The model under review builds one solid part; all positions refer to its coordinate system, in mm. Give positions to 0.01 mm unless a question says otherwise; leave off trailing zeros. Loops run counter-clockwise (first coordinate to the right, second up) from the corner with the lowest first, then second, coordinate; pieces in that order, holes last. Notation, with made-up numbers: (1.5, -35) -> (60.5, -35) arc R8 cw to (60.5, -31) -> close; hole circle Ø6 at (-16.5, 23.25). An arc over 180 degrees is marked (long way). Write each question's results on one line, items separated by ' | '. Start each with the question number.
Q1. Insertion check: pin 1 Ø1.5 at (y, z) = (61.5, 2.5) entering from -X. The pin has a flat end and moves straight along its axis. Give the tip position at first contact, or say it passes through.
Q2. Mouldability with a two-part tool opening along Y and no side actions: class faces 1 (the face through (44, 0, 4)), 2 (the face through (33.49, 28.45, 3.76)), 3 (the face through (44, 94, 0)) as released by +Y, released by -Y, zero draft, split by the parting line, or undercut.
Q3. We need section B-B (y = 25.4). Write out the cut boundary in (x, z).
Q4. Wall thickness on L1, parallel to Y at x = 43.18, z = 6; L2, parallel to X at y = 16.5, z = 7: over which ranges is each line inside the solid? List them lowest first. Write a range as [from, to].
Q5. We need section C-C (z = 1.5). Write out the cut boundary in (x, y), plus the area to 3 significant figures.
Q6. We need section A-A (x = 43.18). Write out the cut boundary in (y, z), plus the area to 3 significant figures.
from build123d import *

# Parameters (mm, degrees)
F0_W     = 88.9
F0_H     = 185.42
F1_DEPTH = 7.62
F3_D     = 20.32


with BuildPart() as f1:
    # F0 (on Top) → F1 (new body)
    with BuildSketch(Plane.XY):
        with Locations((44.45, 92.71)):
            Rectangle(F0_W, F0_H)
    extrude(amount=F1_DEPTH)

    # F3 (through all)
    with Locations(Plane.XY.offset(7.62)):
        with Locations((43.18, 160.02), (43.18, 25.4)):
            Hole(F3_D / 2)


solid = f1.part
Output:
1) pin 1: x = 0
2) face 1: released by -Y | face 2: undercut | face 3: zero draft
3) outline: (0, 0) -> (33.02, 0) -> (33.02, 7.62) -> (0, 7.62) -> close; (53.34, 0) -> (88.9, 0) -> (88.9, 7.62) -> (53.34, 7.62) -> close
4) L1: [0, 15.24], [35.56, 149.86], [170.18, 185.42] | L2: [0, 38.28], [48.08, 88.9]
5) outline: (0, 0) -> (88.9, 0) -> (88.9, 185.42) -> (0, 185.42) -> close; hole circle Ø20.32 at (43.18, 25.4); hole circle Ø20.32 at (43.18, 160.02) | area: 15,800 mm2
6) outline: (0, 0) -> (15.24, 0) -> (15.24, 7.62) -> (0, 7.62) -> close; (35.56, 0) -> (149.86, 0) -> (149.86, 7.62) -> (35.56, 7.62) -> close; (170.18, 0) -> (185.42, 0) -> (185.42, 7.62) -> (170.18, 7.62) -> close | area: 1,100 mm2
